Source: CAD feature listing. Evaluate the final solid. Frame: model axes, mm. A direction names the side the tool comes from. Round coordinates to 2 decimals unless told otherwise and drop trailing zeros. Write each loop counter-clockwise with the first axis right and the second up, starting at its lowest first coordinate (ties: lowest second). Pieces come first, ordered by that corner, then holes. Notation, with made-up numbers: M 54.25,23 L 68.25,23 A5 ccw 68.25,28 Z; hole C 74.25,22 d11. An arc over 180 degrees is marked long. Answer in a Markdown table with one row per item.
from build123d import *

# Parameters (mm, degrees)
SKETCH2_R           = 1.45
BOSS_EXTRUDE1_DEPTH = 10
BOSS_EXTRUDE2_START = 10
SKETCH3_R           = 1.45
BOSS_EXTRUDE2_DEPTH = 10


with BuildPart() as part:
    # Sketch1 → Revolve1 (revolve)
    with BuildSketch(Plane(origin=(0, 0, 0), x_dir=(1, 0, 0), z_dir=(0, 1, 0))):
        with BuildLine():
            Line((0, 0), (0, 46))
            Line((0, 46), (7, 46))
            ThreePointArc((7, 46), (5.226178525, 23), (7, 0))
            Line((7, 0), (0, 0))
        make_face()
    revolve(axis=Axis((0, 0, 0), (0, 0, -1)))

    # Sketch2 → Boss-Extrude1 (add)
    with BuildSketch(Plane.XY):
        Circle(SKETCH2_R)
    extrude(amount=BOSS_EXTRUDE1_DEPTH)

    # Sketch3 → Boss-Extrude2 (add)
    with BuildSketch(Plane(origin=(0, 0, -46), x_dir=(-1, 0, 0), z_dir=(0, 0, -1)).offset(BOSS_EXTRUDE2_START)):
        with Locations(Location((0, 0, 0), (0, 0, 180))):
            Circle(SKETCH3_R)
    extrude(amount=-BOSS_EXTRUDE2_DEPTH)


solid = part.part
Q1. Section C-C (z = -48.5). Return loops of the section in (x, y).
Solutions:
| item | result |
|---|---|
| outline | C 0,0 d2.9 |
Q2. Section D-D (z = -40). Return loops of the section in (x, y).
Solutions:
| item | result |
|---|---|
| outline | C 0,0 d12.39 |
Q3. Material intervals for probe 1 along Z at (x, y) = (4, 2.5); probe 2 along X at (y, z) = (3.25, -1.5); probe 3 along Y at (x, z) = (-5.5, -38.5), sorted ascending.
Solutions:
| item | result |
|---|---|
| probe 1 | z = -46 to 0 |
| probe 2 | x = -5.94 to 5.94 |
| probe 3 | y = -2.47 to 2.47 |
Q4. Access query for faces 1 (the cylindrical face through (1.38, -0.44, -51.07)), 2 (the flat face through (0, 0, -56)), 3 (the cylindrical face through (-1.45, 0.06, 4.93)). Directions: +Z, -Z, +X, -X, +Y, -Y. A direction counts if a zero-diameter tool reaches every point of the face in a straight line with its end or side. Return the directions, or none.
Solutions:
| item | result |
|---|---|
| face 1 | -Z |
| face 2 | -Z, +X, -X, +Y, -Y |
| face 3 | +Z |
Q5. Contact query for flat-ended pins moving along their axis: pin 1 Ø5 at (x, z) = (-2.5, -15) entering from -Y; pin 2 Ø5 at (y, z) = (-0.5, -20.5) entering from +X; pin 3 Ø1.5 at (x, z) = (-4.5, -40.5) entering from -Y. Output: stop coordinate, or through.
Solutions:
| item | result |
|---|---|
| pin 1 | stops at y = -5.5 |
| pin 2 | stops at x = 5.31 |
| pin 3 | stops at y = -5.01 |
Q6. Section A-A (x = 0). Return loops of the section in (y, z), and give its area (3 significant figures).
Solutions:
| item | result |
|---|---|
| outline | M -7,-46 L -1.45,-46 L -1.45,-56 L 1.45,-56 L 1.45,-46 L 7,-46 A150 cw 7,0 L 1.45,0 L 1.45,10 L -1.45,10 L -1.45,0 L -7,0 A150 cw Z |
| area | 593 mm2 |
